Can you work these out from the model? Positions are in its coordinate system, mm. Round coordinates to 2 decimals unless told otherwise and drop trailing zeros. Order: outer loops, then holes, each group sorted by start corner. A loop starts at its lowest first (then second) coordinate and runs counter-clockwise, first axis right, second up. Notation, with made-up numbers: (22.5, 20) -> (43.5, 20) arc R18 cw to (43.5, 32) -> close; hole circle Ø6 at (-37, 41). An arc over 180 degrees is marked (long way). Use a Markdown table: item, result. Add a question column.
Q1. If we section it at A-A on y = 0: List the corners of the cut face in (x, z) for me, plus the area to 3 significant figures.
Q2. I need wall thicknesses on line 1 along Y through (x, z) = (-18, 1.45); line 2 along X through (y, z) = (2, 0.4); line 3 along Y through (x, z) = (18.5, 0.8). Which ranges of each line are inside material? Lowest first, please. Write a range as [from, to].
Q3. If we section it at C-C on y = -36: List the corners of the cut face in (x, z) for me, plus the area to 3 significant figures.
Q4. If we section it at B-B on z = 0.5: Give the number of separate pieces and of enclosed holes in the cut face, plus the area to 3 significant figures.
Q5. I'm going to push a flat-ended pin straight in: pin 1 Ø8 at (x, y) = (30.26, 17.4) entering from +Z. Where does the tip first touch, or does it pass through?
Q6. If we section it at D-D on x = 0: List the corners of the cut face in (y, z) for me.
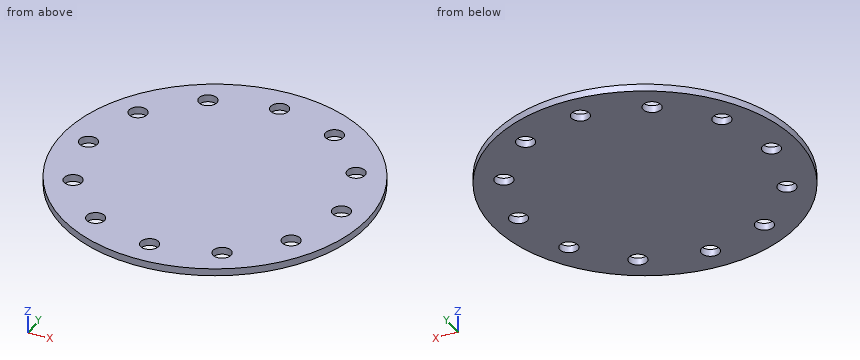
```python
from build123d import *

# Parameters (mm, degrees)
F0_R     = 42.5
F0_R_2   = 2.5
F1_DEPTH = 2


with BuildPart() as f1:
    # F0 (on Top) → F1 (new body)
    with BuildSketch(Plane.XY):
        Circle(F0_R)
        with Locations((-0.220217, -35)):
            Circle(F0_R_2, mode=Mode.SUBTRACT)
        with Locations((-17.555054, -30.406246)):
            Circle(F0_R_2, mode=Mode.SUBTRACT)
        with Locations((-30.476052, -17.404643)):
            Circle(F0_R_2, mode=Mode.SUBTRACT)
        with Locations((17.555054, -30.406246)):
            Circle(F0_R_2, mode=Mode.SUBTRACT)
        with Locations((30.145726, -17.595357)):
            Circle(F0_R_2, mode=Mode.SUBTRACT)
        with Locations((-35.110109, 0)):
            Circle(F0_R_2, mode=Mode.SUBTRACT)
        with Locations((-30.365943, 17.595357)):
            Circle(F0_R_2, mode=Mode.SUBTRACT)
        with Locations((-17.555054, 30.406246)):
            Circle(F0_R_2, mode=Mode.SUBTRACT)
        with Locations((35.110109, 0)):
            Circle(F0_R_2, mode=Mode.SUBTRACT)
        with Locations((30.255835, 17.404643)):
            Circle(F0_R_2, mode=Mode.SUBTRACT)
        with Locations((17.555054, 30.406246)):
            Circle(F0_R_2, mode=Mode.SUBTRACT)
        with Locations((0, 35)):
            Circle(F0_R_2, mode=Mode.SUBTRACT)
    extrude(amount=F1_DEPTH)


solid = f1.part
```
Answer below:
| question | item | result |
|---|---|---|
| 1 | outline | (-42.5, 0) -> (-37.61, 0) -> (-37.61, 2) -> (-42.5, 2) -> close; (-32.61, 0) -> (32.61, 0) -> (32.61, 2) -> (-32.61, 2) -> close; (37.61, 0) -> (42.5, 0) -> (42.5, 2) -> (37.61, 2) -> close |
| 1 | area | 150 mm² |
| 2 | line 1 | [-38.5, -32.87], [-27.95, 27.95], [32.87, 38.5] |
| 2 | line 2 | [-42.45, -36.61], [-33.61, 33.61], [36.61, 42.45] |
| 2 | line 3 | [-38.26, -32.72], [-28.09, 28.09], [32.72, 38.26] |
| 3 | outline | (-22.59, 0) -> (-2.51, 0) -> (-2.51, 2) -> (-22.59, 2) -> close; (2.07, 0) -> (22.59, 0) -> (22.59, 2) -> (2.07, 2) -> close |
| 3 | area | 81.2 mm² |
| 4 | separate pieces | 1 |
| 4 | enclosed holes | 12 |
| 4 | area | 5,440 mm² |
| 5 | pin 1 | z = 2 |
| 6 | outline | (-42.5, 0) -> (-37.49, 0) -> (-37.49, 2) -> (-42.5, 2) -> close; (-32.51, 0) -> (32.5, 0) -> (32.5, 2) -> (-32.51, 2) -> close; (37.5, 0) -> (42.5, 0) -> (42.5, 2) -> (37.5, 2) -> close |
